The listing builds one solid part. Answer for the finished solid, in the listing's coordinates (mm). Coordinates: 2 decimals unless noted, no trailing zeros. Order: outer loops, then holes, each group sorted by start corner. A loop starts at its lowest first (then second) coordinate and runs counter-clockwise, first axis right, second up.
Autodesk Inventor part; units mm, degrees
ref_plane "YZ Plane" through (0, 0, 0) normal (1, 0, 0) x (0, 1, 0)
ref_plane "XZ Plane" through (0, 0, 0) normal (0, 1, 0) x (-1, 0, 0)
ref_plane "XY Plane" through (0, 0, 0) normal (0, 0, 1) x (1, 0, 0)
sketch "Sketch1" plane through (0, 0, 0) normal (0, 0, 1) x (1, 0, 0)
  circle A0 centre (0, 0) radius 30
  circle A1 centre (0, 0) radius 32.5
  dimension "d0" = 60
  dimension "d1" = 2.5
extrude "Extrusion1" add sketch "Sketch1" along normal blind 0.1
sketch "Sketch2" plane through (0, 0, 0.1) normal (0, 0, 1) x (1, 0, 0)
  circle A0 centre (0, 31.25) radius 1
  circle A1 centre (0, 0) radius 32.5
  circle A2 centre (31.25, 0) radius 1
  circle A3 centre (-31.25, 0) radius 1
  circle A4 centre (-0.0425, -31.25) radius 1
  dimension "d4" = 2
  dimension "d5" = 0.25
  dimension "d6" = 2
  dimension "d7" = 0.25
  dimension "d8" = 2
  dimension "d9" = 0.25
  dimension "d10" = 2
  dimension "d11" = 0.25
extrude "Extrusion2" cut sketch "Sketch2" against normal blind 0.2 contours A0 | A2 | A3 | A4
properties part number "cage_electrode"
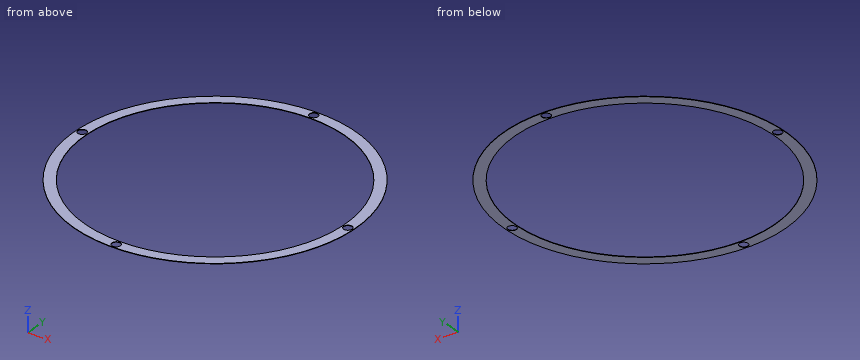
(1) Find section B-B (x = -6.5). Write down the section's boundary in (y, z), and give its area (3 significant figures).
(2) This flat-tipped pin is pushed along its axis until it touches: pin 1 Ø1.8 at (x, y) = (-31.25, 0) entering from +Z. Where does it stop, or does it pass through?
(3) Find section A-A (y = 2.5). Write down the section's boundary in (x, z).
(4) Find section C-C (x = 0). Write down the section's boundary in (y, z).
(5) Consider line 1 (Y direction, x = 0, z = 0.05); line 2 (Y direction, x = -2.5, z = 0.05); line 3 (X direction, y = 1.5, z = 0.05). Determine where each line is inside the solid, lowest interval first.
Findings below:
1. outline: (-31.84, 0) - (-29.29, 0) - (-29.29, 0.1) - (-31.84, 0.1) - close; (29.29, 0) - (31.84, 0) - (31.84, 0.1) - (29.29, 0.1) - close
1. area: 0.511 mm2
2. pin 1: passes through
3. outline: (-32.4, 0) - (-29.9, 0) - (-29.9, 0.1) - (-32.4, 0.1) - close; (29.9, 0) - (32.4, 0) - (32.4, 0.1) - (29.9, 0.1) - close
4. outline: (-32.5, 0) - (-32.25, 0) - (-32.25, 0.1) - (-32.5, 0.1) - close; (-30.25, 0) - (-30, 0) - (-30, 0.1) - (-30.25, 0.1) - close; (30, 0) - (30.25, 0) - (30.25, 0.1) - (30, 0.1) - close; (32.25, 0) - (32.5, 0) - (32.5, 0.1) - (32.25, 0.1) - close
5. line 1: y = -32.5 to -32.25, -30.25 to -30, 30 to 30.25, 32.25 to 32.5
5. line 2: y = -32.4 to -29.9, 29.9 to 32.4
5. line 3: x = -32.47 to -29.96, 29.96 to 32.47
